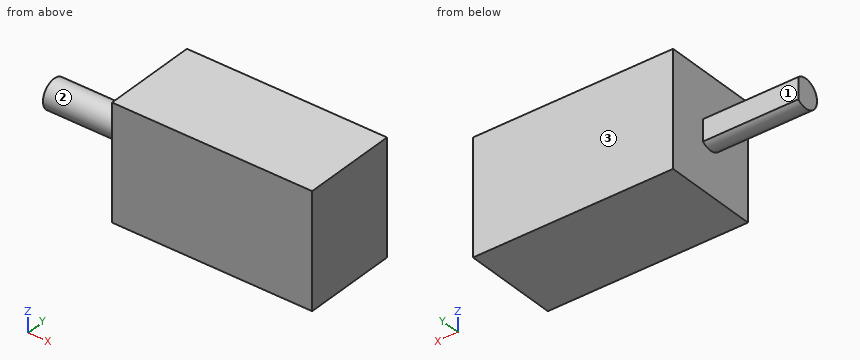
```python
from build123d import *

# Parameters (mm, degrees)
SKETCH1_W           = 21
SKETCH1_H           = 12
BOSS_EXTRUDE1_DEPTH = 10
BOSS_EXTRUDE2_DEPTH = 10


with BuildPart() as part:
    # Sketch1 → Boss-Extrude1 (new body)
    with BuildSketch(Plane(origin=(0, 0, 0), x_dir=(1, 0, 0), z_dir=(0, 1, 0))):
        with Locations((10.5, 6)):
            Rectangle(SKETCH1_W, SKETCH1_H)
    extrude(amount=BOSS_EXTRUDE1_DEPTH)

    # Sketch2 → Boss-Extrude2 (add)
    with BuildSketch(Plane.ZY):
        with BuildLine():
            Line((-7.118033989, 6), (-4.881966011, 6))
            ThreePointArc((-4.881966011, 6), (-6, 3.5), (-7.118033989, 6))
        make_face()
    extrude(amount=BOSS_EXTRUDE2_DEPTH)


solid = part.part
```
Can you work these out from the model? Positions are in its coordinate system, mm. Face numbers are marked on the shaded views. A direction names the side the tool comes from. Coordinates: 2 decimals unless noted, no trailing zeros. Loops run counter-clockwise (first coordinate to the right, second up) from the corner with the lowest first, then second, coordinate; pieces in that order, holes last. Notation, with made-up numbers: (-5.75, 25) -> (45.25, 25) arc R19 cw to (45.25, 34) -> close; hole circle Ø7 at (28.25, 63.25). An arc over 180 degrees is marked (long way). Answer as a JSON object with one key per item and string values.
1) Imagine slicing it at B-B (z = -6). Please give me the cut outline in (x, y).
Results:
{"outline": "(-10, 3.5) -> (0, 3.5) -> (0, 0) -> (21, 0) -> (21, 10) -> (0, 10) -> (0, 6) -> (-10, 6) -> close"}
2) Imagine slicing it at A-A (y = 5). Please give me the cut outline in (x, z).
Results:
{"outline": "(-10, -7.5) -> (0, -7.5) -> (0, -12) -> (21, -12) -> (21, 0) -> (0, 0) -> (0, -4.5) -> (-10, -4.5) -> close"}
3) For P1, Ø2.5, axis at x = -2.5, z = -6.5, coming from the +Y side; P2, Ø5, axis at y = 7.5, z = -9, coming from the -X side; P3, Ø3, axis at x = -2, y = 5, coming from the +Z side; P4, Ø2, axis at y = 5, z = -2.5, coming from the -X side, each with a flat end and sliding along its axis, tell me the tip position at first contact or that it passes through.
Results:
{"P1": "stops at y = 6", "P2": "stops at x = -10", "P3": "stops at z = -4.5", "P4": "stops at x = 0"}
4) If I drill on line 1 (X direction, y = 6.75, z = -5); line 2 (Z direction, x = -7.5, y = 4.25); line 3 (Z direction, x = -7, y = 4.5), over which ranges is the centre line in solid material (lowest first)?
Results:
{"line 1": "x = 0 to 21", "line 2": "z = -7.3 to -4.7", "line 3": "z = -7.41 to -4.59"}
5) For the marked faces 1, 2 and 3, which set-ups out of +Z, -Z, +X, -X, +Y, -Y let a thin tool reach every point of the face, with its end or its side?
Results:
{"face 1": "+Z, -Z, -X, +Y", "face 2": "-X", "face 3": "+Z, -Z, +X, -X, +Y"}
6) Imagine slicing it at C-C (x = -1). Please give me the cut outline in (y, z), then the cut area to 3 significant figures.
Results:
{"outline": "(6, -7.12) -> (6, -4.88) arc R1.5 ccw (long way) to start", "area": "6.29 mm^2"}
7) Imagine slicing it at D-D (z = -10). Please give me the cut outline in (x, y), then the cut area to 3 significant figures.
Results:
{"outline": "(0, 0) -> (21, 0) -> (21, 10) -> (0, 10) -> close", "area": "210 mm^2"}
